Can you work these out from the model? Positions are in its coordinate system, mm. Face numbers are marked on the shaded views. A direction names the side the tool comes from. Coordinates: 2 decimals unless noted, no trailing zeros. Loops run counter-clockwise (first coordinate to the right, second up) from the corner with the lowest first, then second, coordinate; pieces in that order, holes last. Notation, with made-up numbers: (20, 27.25) -> (48, 27.25) arc R11 cw to (48, 36.25) -> close; hole circle Ø1 at (48.25, 11). An arc over 180 degrees is marked (long way). Put each result on its own line as item: value. Start each with the question number.
Item 1: For the marked faces 1, 2 and 3, which set-ups out of +Z, -Z, +X, -X, +Y, -Y let a thin tool reach every point of the face, with its end or its side?
Item 2: If we section it at B-B on z = -44.5: Please give me the cut outline in (x, y), plus the area to 3 significant figures.
Item 3: If we section it at A-A on z = -21.5: Please give me the cut outline in (x, y).
Item 4: Will these pins go through, and if not, where does the flat tip stop? P1, Ø2.5, axis at y = -1, z = 6, coming from the +X side; P2, Ø4, axis at x = -4, z = -25, coming from the +Y side; P3, Ø1.5, axis at x = 5.5, y = 2.5, coming from the +Z side.
Item 5: Please list where these lines run through material, in increasing order: L1, parallel to Z at x = 1.5, y = -1; L2, parallel to X at y = 0.75, z = 5.5; L3, parallel to X at y = -0.25, z = -41.5. Write a range as from..to.
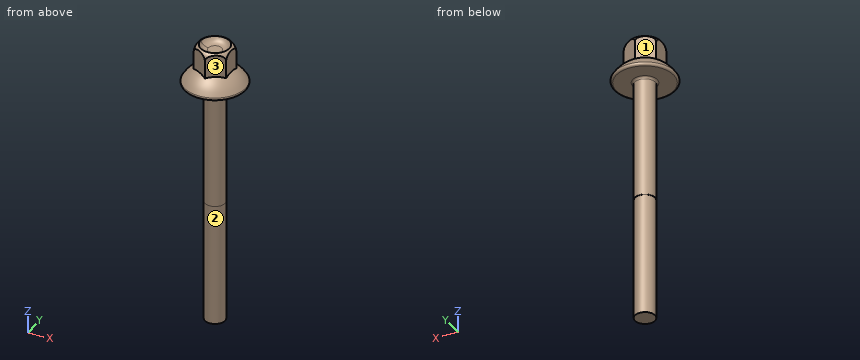
```python
from build123d import *

# Parameters (mm, degrees)
HEAD_DEPTH     = 10
SHANK_SKETCH_R = 2.5
SHANK_DEPTH    = 60
SKETCH6_R      = 3.5
HEAD_CUT_DEPTH = 1.5
FILLET1_R      = 2
FILLET2_R      = 0.5
THREAD_END_W   = 30
THREAD_END_H   = 0.05


with BuildPart() as part:
    # Head Sketch → Head (new body)
    with BuildSketch(Plane.XY):
        Polygon((0, 4.618802154), (4, 2.309401077), (4, -2.309401077), (0, -4.618802154), (-4, -2.309401077), (-4, 2.309401077), align=None)
    extrude(amount=HEAD_DEPTH)

    # Shank Sketch → Shank (add)
    with BuildSketch(Plane.XY):
        Circle(SHANK_SKETCH_R)
    extrude(amount=-SHANK_DEPTH)

    # Sketch3 → Flange (revolve)
    with BuildSketch(Plane(origin=(0, 0, 0), x_dir=(-1, 0, 0), z_dir=(0, 1, 0)), mode=Mode.PRIVATE) as flange_sk:
        with BuildLine():
            Line((-7, 0), (0, 0))
            Line((0, 0), (0, 5))
            ThreePointArc((0, 5), (-4.279198343, 3.863597101), (-7.430769231, 0.753846154))
            ThreePointArc((-7.430769231, 0.753846154), (-7.434121571, 0.251930531), (-7, 0))
        make_face()
    revolve(flange_sk.sketch.rotate(Axis((0, 0, 0), (0, 0, 1)), 30), axis=Axis((0, 0, 0), (0, 0, 1)))

    # Sketch5 → Head Trim (revolve, cut)
    with BuildSketch(Plane(origin=(0, 0, 0), x_dir=(0, 0, -1), z_dir=(1, 0, 0)), mode=Mode.PRIVATE) as head_trim_sk:
        with BuildLine():
            Line((-10, -2.618802154), (-10, -4.618802154))
            Line((-10, -4.618802154), (-8, -4.618802154))
            ThreePointArc((-8, -4.618802154), (-9.414213562, -4.033015716), (-10, -2.618802154))
        make_face()
    revolve(head_trim_sk.sketch.rotate(Axis((0, 0, 15.085599173), (0, 0, -1)), 90), axis=Axis((0, 0, 15.085599173), (0, 0, -1)), mode=Mode.SUBTRACT)

    # Sketch6 → Head Cut (cut)
    with BuildSketch(Plane.XY.offset(10)):
        Circle(SKETCH6_R)
    extrude(amount=-HEAD_CUT_DEPTH, mode=Mode.SUBTRACT)

    # Fillet1
    # the kernel refuses this fillet: 2 mm, written as the material it adds along each edge
    with BuildSketch(Plane(origin=(0, 0, 8.5), x_dir=(1, 0, 0), z_dir=(0, -1, 0))) as fillet1_piece_1:
        with BuildLine():
            CenterArc((1.62822269, 2), FILLET1_R, 270, 69.372190804)
            Line((1.62822269, 0), (3.5, 0))
            Line((3.5, 0), (3.5, 1.295408131))
        make_face()
    revolve(axis=Axis((0, 0, 8.5), (0, 0, 1)), revolution_arc=180.000001341)
    with BuildSketch(Plane(origin=(0, 0, 8.5), x_dir=(-0.9999999999999998, -2.340668935307113e-08, 0), z_dir=(-2.340668935307113e-08, 0.9999999999999998, 0))) as fillet1_piece_2:
        with BuildLine():
            CenterArc((1.62822269, 2), FILLET1_R, 270, 69.372190804)
            Line((1.62822269, 0), (3.5, 0))
            Line((3.5, 0), (3.5, 1.295408131))
        make_face()
    revolve(axis=Axis((0, 0, 8.5), (0, 0, 1)), revolution_arc=179.999998659)

    # Fillet2
    fillet2_edges = [part.edges().sort_by_distance(p)[0] for p in [
        (-2.5, 0, 0),
    ]]
    fillet(fillet2_edges, radius=FILLET2_R)

    # Thread End → Thread Cut (revolve, cut)
    with BuildSketch(Plane(origin=(0, 0, 0), x_dir=(0, 0, -1), z_dir=(1, 0, 0)), mode=Mode.PRIVATE) as thread_cut_sk:
        with Locations((45, 2.475)):
            Rectangle(THREAD_END_W, THREAD_END_H)
    revolve(thread_cut_sk.sketch.rotate(Axis((0, 0, -21.551935625), (0, 0, -1)), 270), axis=Axis((0, 0, -21.551935625), (0, 0, -1)), mode=Mode.SUBTRACT)


solid = part.part
```
Solutions:
1. face 1: +Z, -X, +Y
1. face 2: -Z
1. face 3: +Z, +X, -Y
2. outline: circle Ø4.9 at (0, 0)
2. area: 18.9 mm^2
3. outline: circle Ø5 at (0, 0)
4. P1: x = 4
4. P2: y = 1.5
4. P3: z = 3.19
5. L1: -60..8.51
5. L2: -4..4
5. L3: -2.44..2.44
